from build123d import *

# Parameters (mm, degrees)
SKETCH1_W           = 477.670351936
SKETCH1_H           = 347.715917952
BOSS_EXTRUDE1_DEPTH = 10
CUT_EXTRUDE1_DEPTH  = 10


with BuildPart() as part:
    # Sketch1 → Boss-Extrude1 (new body)
    with BuildSketch(Plane.XY):
        Rectangle(SKETCH1_W, SKETCH1_H)
    extrude(amount=BOSS_EXTRUDE1_DEPTH)

    # Sketch2 → Cut-Extrude1 (cut)
    with BuildSketch(Plane.XY.offset(10)):
        with BuildLine():
            Line((-195.403718463, 65.573687729), (-110.55090472, 150.426501471))
            ThreePointArc((-110.55090472, 150.426501471), (-82.266633473, 150.426501471), (-82.266633473, 122.142230224))
            Line((-82.266633473, 122.142230224), (-167.119447215, 37.289416482))
            ThreePointArc((-167.119447215, 37.289416482), (-195.403718463, 37.289416482), (-195.403718463, 65.573687729))
        make_face()
        with BuildLine():
            Line((38.835175968, 133.857958976), (178.835175968, 133.857958976))
            ThreePointArc((178.835175968, 133.857958976), (198.835175968, 113.857958976), (178.835175968, 93.857958976))
            Line((178.835175968, 93.857958976), (38.835175968, 93.857958976))
            ThreePointArc((38.835175968, 93.857958976), (18.835175968, 113.857958976), (38.835175968, 133.857958976))
        make_face()
        with BuildLine():
            ThreePointArc((21.164824032, -113.857958976), (-98.835175968, 6.142041024), (-218.835175968, -113.857958976))
            ThreePointArc((-218.835175968, -113.857958976), (-198.835175968, -133.857958976), (-178.835175968, -113.857958976))
            ThreePointArc((-178.835175968, -113.857958976), (-98.835175968, -33.857958976), (-18.835175968, -113.857958976))
            ThreePointArc((-18.835175968, -113.857958976), (1.164824032, -133.857958976), (21.164824032, -113.857958976))
        make_face()
        with BuildLine():
            ThreePointArc((186.889668623, 60.453082732), (118.835175968, 33.988137932), (61.888615133, -11.716309149))
            ThreePointArc((61.888615133, -11.716309149), (63.122357717, -39.973660037), (91.379708606, -38.739917453))
            ThreePointArc((91.379708606, -38.739917453), (138.835175968, -0.65287822), (195.54725318, 21.401242448))
            ThreePointArc((195.54725318, 21.401242448), (210.744381044, 45.255954869), (186.889668623, 60.453082732))
        make_face()
    extrude(amount=-CUT_EXTRUDE1_DEPTH, mode=Mode.SUBTRACT)


solid = part.part
CAD build for the part. Positions are in the model's coordinates, mm. A direction names the side the tool comes from. Round coordinates to 2 decimals unless told otherwise and drop trailing zeros. Loops run counter-clockwise (first coordinate to the right, second up) from the corner with the lowest first, then second, coordinate; pieces in that order, holes last. Notation, with made-up numbers: (-2.5, -29) - (18.5, -29) arc R10 ccw to (18.5, -11) - close; hole circle Ø3 at (36, 78). An arc over 180 degrees is marked (long way). Put each result on its own line as item: value.
1. Slice it at B-B on x = 135. List the corners of the cut face in (y, z), and give its area (3 significant figures).
Geometry check:
outline: (-173.86, 0) - (-2.92, 0) - (-2.92, 10) - (-173.86, 10) - close; (42.52, 0) - (93.86, 0) - (93.86, 10) - (42.52, 10) - close; (133.86, 0) - (173.86, 0) - (173.86, 10) - (133.86, 10) - close
area: 2,620 mm²
2. Two-plate mould, pull along Y, no slides. Class faces 1 (the cylindrical face through (-199.275, -133.853, 5.07)), 2 (the flat face through (-3, 173.858, 5)), 3 (the flat face through (238.835, -2, 5)): released by +Y, released by -Y, zero draft, split by the parting line, or undercut.
Geometry check:
face 1: undercut
face 2: released by +Y
face 3: zero draft
3. Slice it at A-A on z = 6.5. List the corners of the cut face in (x, y).
Geometry check:
outline: (-238.84, -173.86) - (238.84, -173.86) - (238.84, 173.86) - (-238.84, 173.86) - close; hole (-218.84, -113.86) arc R20 ccw to (-178.84, -113.86) arc R80 cw to (-18.84, -113.86) arc R20 ccw to (21.16, -113.86) arc R120 ccw to start; hole (-195.4, 65.57) arc R20 ccw to (-167.12, 37.29) - (-82.27, 122.14) arc R20 ccw to (-110.55, 150.43) - close; hole (38.84, 93.86) - (178.84, 93.86) arc R20 ccw to (178.84, 133.86) - (38.84, 133.86) arc R20 ccw to start; hole (61.89, -11.72) arc R20 ccw to (91.38, -38.74) arc R200 cw to (195.55, 21.4) arc R20 ccw to (186.89, 60.45) arc R240 ccw to start
4. Slice it at D-D on y = 77. List the corners of the cut face in (x, z), and give its area (3 significant figures).
Geometry check:
outline: (-238.84, 0) - (-183.98, 0) - (-183.98, 10) - (-238.84, 10) - close; (-127.41, 0) - (238.84, 0) - (238.84, 10) - (-127.41, 10) - close
area: 4,210 mm²
5. Wall check: line 1 (Y direction, x = 55.5, z = 8); line 2 (Y direction, x = 145, z = 1.5); line 3 (Y direction, x = -149, z = 8.25). Give the ranges that are in metal, low to high.
Geometry check:
line 1: -173.86 to 93.86, 133.86 to 173.86
line 2: -173.86 to 2.76, 47.04 to 93.86, 133.86 to 173.86
line 3: -173.86 to -51.54, -4.85 to 55.41, 111.98 to 173.86
6. 3-axis set-ups, long thin cutter, end or side, ignore diameter. For faces 4 (the cylindrical face through (-100.594, -33.877, 5.07)), 5 (the flat face through (-3, 2, 10)): which of +Z, -Z, +X, -X, +Y, -Y reach the whole face in a straight line?
Geometry check:
face 4: +Z, -Z
face 5: +Z, +X, -X, +Y, -Y
7. Slice it at C-C on x = -12.5. List the corners of the cut face in (y, z), and give its area (3 significant figures).
Geometry check:
outline: (-173.86, 0) - (-128.46, 0) - (-128.46, 10) - (-173.86, 10) - close; (-30.51, 0) - (173.86, 0) - (173.86, 10) - (-30.51, 10) - close
area: 2,500 mm²
